Part model, mm, in its own coordinate system. Face numbers are marked on the shaded views. A direction names the side the tool comes from. Round coordinates to 2 decimals unless told otherwise and drop trailing zeros. Loops run counter-clockwise (first coordinate to the right, second up) from the corner with the lowest first, then second, coordinate; pieces in that order, holes last.
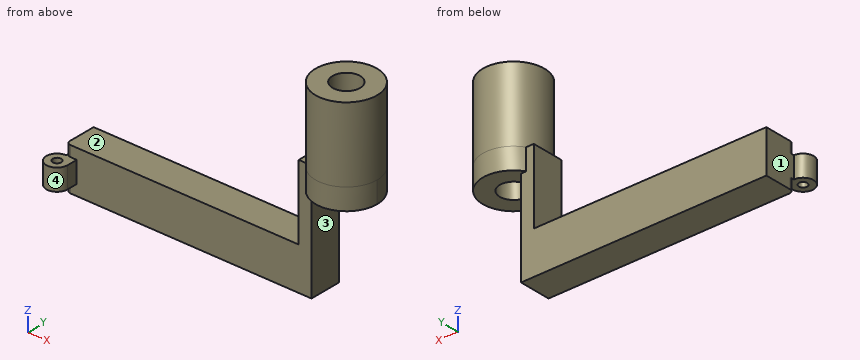
from build123d import *

# Parameters (mm, degrees)
SKETCH4_W                = 20
SKETCH4_H                = 15
BOSS_EXTRUDE1_DEPTH      = 115.8
SKETCH5_W                = 6
SKETCH5_H                = 15
BOSS_EXTRUDE2_DEPTH      = 35
SKETCH6_R                = 14.5
SKETCH6_R_2              = 6.5
BOSS_EXTRUDE3_DEPTH      = 35
BOSS_EXTRUDE3_DEPTH_BACK = 10
SKETCH7_R                = 2
BOSS_EXTRUDE4_DEPTH      = 5
FILLET1_R                = 2


with BuildPart() as part:
    # Sketch4 → Boss-Extrude1 (new body)
    with BuildSketch(Plane(origin=(0, 0, 0), x_dir=(0, 0, -1), z_dir=(1, 0, 0))):
        Rectangle(SKETCH4_W, SKETCH4_H)
    extrude(amount=BOSS_EXTRUDE1_DEPTH)

    # Sketch5 → Boss-Extrude2 (add)
    with BuildSketch(Plane.XY.offset(10)):
        with Locations((112.8, 0)):
            Rectangle(SKETCH5_W, SKETCH5_H)
    extrude(amount=BOSS_EXTRUDE2_DEPTH)

    # Sketch6 → Boss-Extrude3 (add, two sides)
    with BuildSketch(Plane.XY.offset(45)) as boss_extrude3_sk:
        with Locations((125.8, 0)):
            Circle(SKETCH6_R)
        with Locations((125.8, 0)):
            Circle(SKETCH6_R_2, mode=Mode.SUBTRACT)
    extrude(amount=BOSS_EXTRUDE3_DEPTH)
    extrude(boss_extrude3_sk.sketch, amount=-BOSS_EXTRUDE3_DEPTH_BACK)

    # Sketch7 → Boss-Extrude4 (add, symmetric)
    with BuildSketch(Plane.XY):
        with BuildLine():
            Line((5, -12.5), (5, -7.5))
            Line((5, -7.5), (0, -7.5))
            ThreePointArc((0, -7.5), (-3.535533906, -16.035533906), (5, -12.5))
        make_face()
        with Locations((0, -12.5)):
            Circle(SKETCH7_R, mode=Mode.SUBTRACT)
    extrude(amount=BOSS_EXTRUDE4_DEPTH, both=True)

    # Fillet1
    fillet1_edges = [part.edges().sort_by_distance(p)[0] for p in [
        (0, -7.5, -7.5),
        (0, -7.5, 7.5),
    ]]
    fillet(fillet1_edges, radius=FILLET1_R)


solid = part.part
1) Wall check: line 1 along Y through (x, z) = (125.8, 40.5); line 2 along X through (y, z) = (-6, 69.5); line 3 along Y through (x, z) = (105.5, -5.5). Give the ranges that are in metal, low to high.
Values:
line 1: y = -14.5 to -6.5, 6.5 to 14.5
line 2: x = 112.6 to 123.3, 128.3 to 139
line 3: y = -7.5 to 7.5
2) Drop flat-ended pins along their axis: pin 1 Ø6 at (x, y) = (24, -9) entering from +Z; pin 2 Ø16.5 at (y, z) = (1.5, -2) entering from -X; pin 3 Ø4.5 at (y, z) = (-1.5, 23.5) entering from -X. Give the stop position or say it passes through.
Values:
pin 1: stops at z = 10
pin 2: stops at x = 0
pin 3: stops at x = 109.8
3) Tool access for the marked faces 1, 2, 3 and 4: list every direction of +Z, -Z, +X, -X, +Y, -Y with a clear straight run to the whole face (end or side of a thin tool).
Values:
face 1: +Z, -Z, -X, +Y
face 2: +Z, -X, +Y, -Y
face 3: -Z, +X, +Y, -Y
face 4: +Z, -Z
4) Slice it at D-D, the plane z = 24. Give the cut face in (x, y).
Values:
outline: (109.8, -7.5) - (115.8, -7.5) - (115.8, 7.5) - (109.8, 7.5) - close
5) Slice it at A-A, the plane x = 125.8. Give the cut face in (y, z).
Values:
outline: (-14.5, 35) - (-6.5, 35) - (-6.5, 80) - (-14.5, 80) - close; (6.5, 35) - (14.5, 35) - (14.5, 80) - (6.5, 80) - close
6) Slice it at C-C, the plane z = 40.5. Give the cut face in (x, y), then the cut area to 3 significant figures.
Values:
outline: (109.8, -7.5) - (113.39, -7.5) arc R14.5 ccw (long way) to (113.39, 7.5) - (109.8, 7.5) - close; hole circle Ø13 at (125.8, 0)
area: 560 mm2
7) Slice it at B-B, the plane y = 2. Give the cut face in (x, z), then the cut area to 3 significant figures.
Values:
outline: (0, -10) - (115.8, -10) - (115.8, 35) - (119.62, 35) - (119.62, 80) - (111.44, 80) - (111.44, 45) - (109.8, 45) - (109.8, 10) - (0, 10) - close; (131.98, 35) - (140.16, 35) - (140.16, 80) - (131.98, 80) - close
area: 3,220 mm2
